Can you work these out from the model? Positions are in its coordinate system, mm. A direction names the side the tool comes from. Round coordinates to 2 decimals unless told otherwise and drop trailing zeros. Loops run counter-clockwise (first coordinate to the right, second up) from the corner with the lowest first, then second, coordinate; pieces in that order, holes last. Notation, with made-up numbers: (-13.5, 62) -> (3.5, 62) arc R38 cw to (3.5, 100) -> close; hole circle Ø8 at (-8.75, 23.25). An arc over 180 degrees is marked (long way). Answer as a JSON object with one key per item and string values.
```python
from build123d import *

# Parameters (mm, degrees)
SKETCH1_R           = 2.54
SKETCH1_W           = 31.75
SKETCH1_H           = 5.08
BOSS_EXTRUDE1_DEPTH = 5.08


with BuildPart() as part:
    # Sketch1 → Boss-Extrude1 (new body)
    with BuildSketch(Plane.XY):
        with BuildLine():
            Line((73.443857446, 124.317776281), (22.310144528, 124.317776281))
            Line((22.310144528, 124.317776281), (22.310144528, 129.397776281))
            Line((22.310144528, 129.397776281), (14.0979145, 129.397776281))
            Line((14.0979145, 129.397776281), (-30.3520855, 129.397776281))
            Line((-30.3520855, 129.397776281), (-36.559880198, 129.397776281))
            Line((-36.559880198, 129.397776281), (-36.559880198, 124.317776281))
            Line((-36.559880198, 124.317776281), (-87.693593116, 124.317776281))
            Line((-87.693593116, 124.317776281), (-87.693593116, 129.397776281))
            Line((-87.693593116, 129.397776281), (-96.342075919, 129.397776281))
            ThreePointArc((-96.342075919, 129.397776281), (-101.730229592, 127.165929953), (-103.962075919, 121.777776281))
            Line((-103.962075919, 121.777776281), (-98.882075919, 121.777776281))
            Line((-98.882075919, 121.777776281), (-98.882075919, 56.048326859))
            Line((-98.882075919, 56.048326859), (-103.962075919, 56.048326859))
            ThreePointArc((-103.962075919, 56.048326859), (-101.730229592, 50.660173186), (-96.342075919, 48.428326859))
            Line((-96.342075919, 48.428326859), (-87.693593116, 48.428326859))
            Line((-87.693593116, 48.428326859), (-87.693593116, 53.508326859))
            Line((-87.693593116, 53.508326859), (-58.190357776, 53.508326859))
            Line((-58.190357776, 53.508326859), (-58.190357776, 48.428326859))
            Line((-58.190357776, 48.428326859), (-45.221913897, 48.428326859))
            Line((-45.221913897, 48.428326859), (-45.221913897, 0.116289741))
            Line((-45.221913897, 0.116289741), (-7.123980427, 0.116289741))
            Line((-7.123980427, 0.116289741), (15.101019573, 0.116289741))
            Line((15.101019573, 0.116289741), (15.101019573, 48.428326859))
            Line((15.101019573, 48.428326859), (32.202561113, 48.428326859))
            Line((32.202561113, 48.428326859), (43.940622107, 48.428326859))
            Line((43.940622107, 48.428326859), (43.940622107, 53.508326859))
            Line((43.940622107, 53.508326859), (73.443857446, 53.508326859))
            Line((73.443857446, 53.508326859), (73.443857446, 48.428326859))
            Line((73.443857446, 48.428326859), (80.087904918, 48.428326859))
            ThreePointArc((80.087904918, 48.428326859), (85.476058591, 50.660173186), (87.707904918, 56.048326859))
            Line((87.707904918, 56.048326859), (82.627904918, 56.048326859))
            Line((82.627904918, 56.048326859), (82.627904918, 116.106668145))
            Line((82.627904918, 116.106668145), (82.627904918, 121.777776281))
            Line((82.627904918, 121.777776281), (87.707904918, 121.777776281))
            ThreePointArc((87.707904918, 121.777776281), (85.476058591, 127.165929953), (80.087904918, 129.397776281))
            Line((80.087904918, 129.397776281), (73.443857446, 129.397776281))
            Line((73.443857446, 129.397776281), (73.443857446, 124.317776281))
        make_face()
        Polygon((-3.872275334, 3.339373144), (-39.506956929, 3.339373144), (-39.506956929, 11.703040428), (-3.872275334, 10.997950476), align=None, mode=Mode.SUBTRACT)
        with Locations((-63.737543347, 63.552037118)):
            Circle(SKETCH1_R, mode=Mode.SUBTRACT)
        Polygon((-39.506956929, 39.861286156), (-29.349867835, 39.861286156), (-3.872275334, 39.861286156), (-3.872275334, 33.84416171), (-39.506956929, 33.84416171), align=None, mode=Mode.SUBTRACT)
        with Locations((-7.123980427, 50.968326859)):
            Rectangle(SKETCH1_W, SKETCH1_H, mode=Mode.SUBTRACT)
        with Locations((-7.124867835, 61.012037118)):
            Rectangle(SKETCH1_W, SKETCH1_H, mode=Mode.SUBTRACT)
        with Locations((49.487807678, 63.552037118)):
            Circle(SKETCH1_R, mode=Mode.SUBTRACT)
        with Locations((-63.737543347, 113.231437191)):
            Circle(SKETCH1_R, mode=Mode.SUBTRACT)
        with BuildLine():
            Line((70.649018329, 71.162232039), (-84.898753999, 71.162232039))
            ThreePointArc((-84.898753999, 71.162232039), (-90.286907671, 73.394078367), (-92.518753999, 78.782232039))
            Line((-92.518753999, 78.782232039), (-92.518753999, 92.693311063))
            ThreePointArc((-92.518753999, 92.693311063), (-90.286907671, 98.081464736), (-84.898753999, 100.313311063))
            Line((-84.898753999, 100.313311063), (70.649018329, 100.313311063))
            ThreePointArc((70.649018329, 100.313311063), (76.037172002, 98.081464736), (78.269018329, 92.693311063))
            Line((78.269018329, 92.693311063), (78.269018329, 78.782232039))
            ThreePointArc((78.269018329, 78.782232039), (76.037172002, 73.394078367), (70.649018329, 71.162232039))
        make_face(mode=Mode.SUBTRACT)
        with Locations((-7.124867835, 108.486668145)):
            Rectangle(SKETCH1_W, SKETCH1_H, mode=Mode.SUBTRACT)
        with Locations((-7.124867835, 118.646668145)):
            Rectangle(SKETCH1_W, SKETCH1_H, mode=Mode.SUBTRACT)
        with Locations((49.487807678, 113.231437191)):
            Circle(SKETCH1_R, mode=Mode.SUBTRACT)
    extrude(amount=BOSS_EXTRUDE1_DEPTH)


solid = part.part
```
Q1. I want a section at B-B, the plane y = 82. Write out the boundary of the cut face in (x, z).
Determined:
{"outline": "(-98.88, 0) -> (-92.52, 0) -> (-92.52, 5.08) -> (-98.88, 5.08) -> close; (78.27, 0) -> (82.63, 0) -> (82.63, 5.08) -> (78.27, 5.08) -> close"}
Q2. I want a section at A-A, the plane x = 68.5. Write out the boundary of the cut face in (y, z), then the cut area to 3 significant figures.
Determined:
{"outline": "(53.51, 0) -> (71.16, 0) -> (71.16, 5.08) -> (53.51, 5.08) -> close; (100.31, 0) -> (124.32, 0) -> (124.32, 5.08) -> (100.31, 5.08) -> close", "area": "212 mm²"}
Q3. On a 3-axis mill with a long thin cutter (end or side, diameter ignored), from which of +Z, -Z, +X, -X, +Y, -Y can I reach the whole of each face in a straight line? I mean faces 4 (the flat face through (-101, 121.778, 3)), 5 (the flat face through (82.628, 88, 3)), 6 (the flat face through (78.269, 86, 3)), 7 (the flat face through (48, 124.318, 3)), 8 (the flat face through (58, 53.508, 3)). Say none if no direction works.
Determined:
{"face 4": "+Z, -Z, -X", "face 5": "+Z, -Z, +X", "face 6": "+Z, -Z", "face 7": "+Z, -Z, +Y", "face 8": "+Z, -Z, -Y"}
Q4. I want a section at C-C, the plane x = 0. Write out the boundary of the cut face in (y, z).
Determined:
{"outline": "(0.12, 0) -> (48.43, 0) -> (48.43, 5.08) -> (0.12, 5.08) -> close; (53.51, 0) -> (58.47, 0) -> (58.47, 5.08) -> (53.51, 5.08) -> close; (63.55, 0) -> (71.16, 0) -> (71.16, 5.08) -> (63.55, 5.08) -> close; (100.31, 0) -> (105.95, 0) -> (105.95, 5.08) -> (100.31, 5.08) -> close; (111.03, 0) -> (116.11, 0) -> (116.11, 5.08) -> (111.03, 5.08) -> close; (121.19, 0) -> (129.4, 0) -> (129.4, 5.08) -> (121.19, 5.08) -> close"}
Q5. We'd pull the mould along X, two halves only. Please class faces 1 (the flat face through (85, 121.778, 3)), 2 (the cylindrical face through (-101.79, 50.72, 2.5)), 3 (the flat face through (-7, 116.107, 3)): pulls with the +X half, pulls with the -X half, needs draft (parallel to the pull), parting line crosses it, or undercut.
Determined:
{"face 1": "needs draft", "face 2": "pulls with the -X half", "face 3": "undercut"}
Q6. I'm going to push flat-ended pins straight in: pin 1 (2.5 mm diameter, centred on y = 109.5, z = 3.5, fed in from +X); pin 2 (3 mm diameter, centred on y = 23, z = 2.5, fed in from +X); pin 3 (1 mm diameter, centred on y = 44.5, z = 3.5, fed in from -X). Where does each tip first touch, or does it pass through?
Determined:
{"pin 1": "x = 82.63", "pin 2": "x = 15.1", "pin 3": "x = -45.22"}
Q7. If I drill on L1, parallel to Y at x = -38, z = 2.8; L2, parallel to X at y = 113.5, z = 0.3; L3, parallel to Y at x = 1, z = 1.95, over which ranges is the centre line in solid material (lowest first)? Write a range as [from, to].
Determined:
{"L1": "[0.12, 3.34], [11.67, 33.84], [39.86, 71.16], [100.31, 124.32]", "L2": "[-98.88, -66.26], [-61.21, 46.96], [52.01, 82.63]", "L3": "[0.12, 48.43], [53.51, 58.47], [63.55, 71.16], [100.31, 105.95], [111.03, 116.11], [121.19, 129.4]"}
Q8. I want a section at D-D, the plane z = 2.05. Give the number of separate pieces and of enclosed holes in the cut face, then the cut area to 3 significant figures.
Determined:
{"separate pieces": "1", "enclosed holes": "11", "area": "10,700 mm²"}
